from build123d import *

# Parameters (mm, degrees)
F2_DEPTH = 25
F1_R     = 20
F3_DEPTH = 700
F4_R     = 49.99999


# Not quite as in the source:
# - a fillet or chamfer is up to 0.001 mm smaller than in the source, because OpenCascade refuses the exact size


with BuildPart() as f2:
    # F0 (on Top) → F2 (new body)
    with BuildSketch(Plane.XY):
        Polygon((0, 0), (0, 300), (-346.4101615138, 300), (-692.8203230276, -300), (0, -300), align=None)
        Polygon((346.4101615138, 300), (0, 300), (0, 0), (0, -300), (692.8203230276, -300), align=None)
    extrude(amount=F2_DEPTH)

    # F1 (on Top) → F3 (join)
    with BuildSketch(Plane.XY):
        with Locations((-328.9101615138, 269.6891108675)):
            Circle(F1_R)
        with Locations((-632.1985447626, -265)):
            Circle(F1_R)
        with Locations((328.9101615138, 269.6891108675)):
            Circle(F1_R)
        with Locations((632.1985447626, -265)):
            Circle(F1_R)
    extrude(amount=-F3_DEPTH)

    # F4 (radius 50 in the source; OpenCascade refuses exactly that, so slightly less here)
    f4_edges = [f2.edges().sort_by_distance(p)[0] for p in [
        (-692.820323, -300, 12.5),
        (-346.410162, 300, 12.5),
        (346.410162, 300, 12.5),
        (692.820323, -300, 12.5),
    ]]
    fillet(f4_edges, radius=F4_R)


solid = f2.part
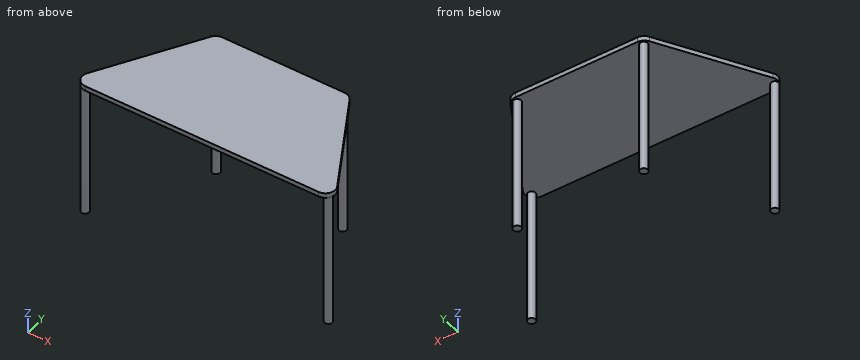
Geometry check sheet. Reference: the model listing, model coordinates, mm. Give positions to 0.01 mm unless a question says otherwise; leave off trailing zeros. Loops run counter-clockwise (first coordinate to the right, second up) from the corner with the lowest first, then second, coordinate; pieces in that order, holes last.
(1) Section check A-A on y = -265. Record the cut outline in (x, z), then the cut area to 3 significant figures.
From the geometry:
outline: (-653.91, 0) - (-652.2, 0) - (-652.2, -700) - (-612.2, -700) - (-612.2, 0) - (612.2, 0) - (612.2, -700) - (652.2, -700) - (652.2, 0) - (653.91, 0) - (653.91, 25) - (-653.91, 25) - close
area: 88,700 mm2
(2) Thickness scan on L1, parallel to Z at x = 444.5, y = -108; L2, parallel to X at y = -249, z = -311.5. Record the ranges inside material, lowest first.
From the geometry:
L1: z = 0 to 25
L2: x = -644.2 to -620.2, 620.2 to 644.2
(3) Section check C-C on x = 24. Record the cut outline in (y, z), then the cut area to 3 significant figures.
From the geometry:
outline: (-300, 0) - (300, 0) - (300, 25) - (-300, 25) - close
area: 15,000 mm2
(4) Section check B-B on z = -86. Record the cut outline in (x, y).
From the geometry:
outline: circle Ø40 at (-632.2, -265); circle Ø40 at (-328.91, 269.69); circle Ø40 at (328.91, 269.69); circle Ø40 at (632.2, -265)
(5) Section check D-D on y = -134. Record the cut outline in (x, z), then the cut area to 3 significant figures.
From the geometry:
outline: (-596.98, 0) - (596.98, 0) - (596.98, 25) - (-596.98, 25) - close
area: 29,800 mm2
(6) Depth check by flat-ended pin: pin 1 Ø6 at (x, y) = (268.5, 113.5) entering from -Z. Enter the tip coordinate at first touch or a pass-through.
From the geometry:
pin 1: stops at z = 0
